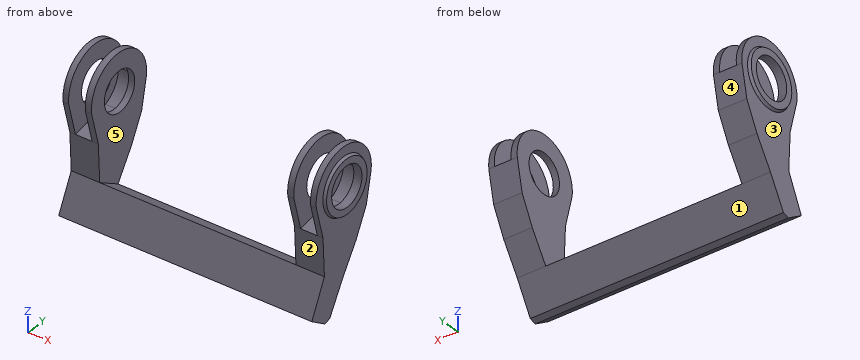
from build123d import *

# Parameters (mm, degrees)
BOSS_EXTRUDE1_DEPTH      = 110.9489018
BOSS_EXTRUDE1_DEPTH_BACK = 110.9489018
BOSS_EXTRUDE2_DEPTH      = 32.209994
CUT_EXTRUDE1_DEPTH       = 18.876772
CUT_EXTRUDE2_DEPTH       = 416.307857918
CUT_EXTRUDE2_DEPTH_BACK  = 416.307857918
SKETCH5_R                = 22.292778643


with BuildPart() as part:
    # Sketch1 → Boss-Extrude1 (new, two sides: drawn at the far end of the back side and taken through both)
    with BuildSketch(Plane(origin=(0, 0, 0), x_dir=(0, 0, -1), z_dir=(1, 0, 0)).offset(-BOSS_EXTRUDE1_DEPTH_BACK)):
        Polygon((6.83514, 301.821342), (21.92401, 328.61631), (55.395622, 309.582058), (57.54243, 302.475138), (45.347128, 283.376878), align=None)
    extrude(amount=BOSS_EXTRUDE1_DEPTH + BOSS_EXTRUDE1_DEPTH_BACK)

    # Sketch2 → Boss-Extrude2 (add)
    with BuildSketch(Plane(origin=(110.9489018, 0, 0), x_dir=(0, 0, -1), z_dir=(1, 0, 0))):
        with BuildLine():
            Line((6.83514, 301.821342), (45.347128, 283.376878))
            Line((45.347128, 283.376878), (57.54243, 302.475138))
            Line((57.54243, 302.475138), (55.395622, 309.582058))
            Line((55.395622, 309.582058), (21.92401, 328.61631))
            Line((21.92401, 328.61631), (-9.123759242, 348.442038748))
            Line((-9.123759242, 348.442038748), (-38.632384, 363.30001))
            Line((-38.632384, 363.30001), (-72.944482, 370.416836))
            ThreePointArc((-72.944482, 370.416836), (-117.407477991, 329.968892479), (-72.634094, 289.8648))
            Line((-72.634094, 289.8648), (-35.4457, 299.743114))
            Line((-35.4457, 299.743114), (6.83514, 301.821342))
        make_face()
    boss_extrude2 = extrude(amount=BOSS_EXTRUDE2_DEPTH)

    # Sketch3 → Cut-Extrude1 (cut)
    with BuildSketch(Plane(origin=(117.9218622, 0, 0), x_dir=(0, 0, -1), z_dir=(1, 0, 0))):
        with BuildLine():
            Line((-72.944482, 370.416836), (-74.851006, 362.67771))
            ThreePointArc((-74.851006, 362.67771), (-56.970321512, 357.844301113), (-44.98594, 343.721436))
            Line((-44.98594, 343.721436), (-35.4457, 299.743114))
            Line((-35.4457, 299.743114), (-71.143283627, 263.85225615))
            Line((-71.143283627, 263.85225615), (-147.020328304, 329.117126747))
            Line((-147.020328304, 329.117126747), (-87.829159197, 385.301513197))
            Line((-87.829159197, 385.301513197), (-72.944482, 370.416836))
        make_face()
    cut_extrude1 = extrude(amount=CUT_EXTRUDE1_DEPTH, mode=Mode.SUBTRACT)

    # Sketch4 → Revolve1 (revolve)
    with BuildSketch(Plane.XY.offset(75.57643), mode=Mode.PRIVATE) as revolve1_sk:
        Polygon((141.481302, 363.150404), (146.090386, 360.588814), (146.090386, 330.870306), (141.481302, 330.870306), align=None)
    revolve1 = revolve(revolve1_sk.sketch.rotate(Axis((146.090386, 330.870306, 75.57643), (-1, 0, 0)), 90), axis=Axis((146.090386, 330.870306, 75.57643), (-1, 0, 0)))

    # Mirror1: Boss-Extrude2, Cut-Extrude1, Revolve1 across plane
    add(boss_extrude2.mirror(Plane(origin=(0, 0, 0), x_dir=(0, 0, 1), z_dir=(1, 0, 0))))
    add(cut_extrude1.mirror(Plane(origin=(0, 0, 0), x_dir=(0, 0, 1), z_dir=(1, 0, 0))), mode=Mode.SUBTRACT)
    add(revolve1.mirror(Plane(origin=(0, 0, 0), x_dir=(0, 0, 1), z_dir=(1, 0, 0))))

    # Sketch5 → Cut-Extrude2 (cut, two sides: drawn at the far end of the back side and taken through both)
    with BuildSketch(Plane(origin=(0, 0, 0), x_dir=(0, 0, -1), z_dir=(1, 0, 0)).offset(-CUT_EXTRUDE2_DEPTH_BACK)):
        with Locations((-75.57643, 330.870306)):
            Circle(SKETCH5_R)
    extrude(amount=CUT_EXTRUDE2_DEPTH + CUT_EXTRUDE2_DEPTH_BACK, mode=Mode.SUBTRACT)


solid = part.part
The model under review builds one solid part; all positions refer to its coordinate system, in mm. Face numbers are marked on the shaded views. A direction names the side the tool comes from. Coordinates: 2 decimals unless noted, no trailing zeros. Loops run counter-clockwise (first coordinate to the right, second up) from the corner with the lowest first, then second, coordinate; pieces in that order, holes last.
(1) Tool access review of the marked faces 1 and 2: name each direction out of +Z, -Z, +X, -X, +Y, -Y from which nothing blocks a thin tool from reaching the whole face with its end or side.
Determined:
face 1: -Z, +X, -X, +Y
face 2: +X, -X, -Y
(2) Insertion check: P1, Ø1, axis at y = 321, z = -32.5, coming from the +X side; P2, Ø4, axis at x = 0, z = -3, coming from the +Y side; P3, Ø8, axis at x = 105, y = 293, coming from the -Z side; P4, Ø1.5, axis at y = 336.5, z = 45.5, coming from the -X side. Each pin has a flat end and moves straight along its axis. Give the tip position at first contact, or say it passes through.
Determined:
P1: stops at x = 143.16
P2: passes through
P3: stops at z = -54.05
P4: stops at x = -145.86
(3) Wall thickness on L1, parallel to X at y = 299, z = 72.5; L2, parallel to X at y = 334.5, z = -2; L3, parallel to X at y = 304, z = 68: over which ranges is each line inside the solid? List them lowest first.
Determined:
L1: x = -143.16 to -136.8, -117.92 to -110.95, 110.95 to 117.92, 136.8 to 143.16
L2: x = -143.16 to -110.95, 110.95 to 143.16
L3: x = -146.09 to -136.8, -117.92 to -110.95, 110.95 to 117.92, 136.8 to 146.09
(4) Draft analysis for pull direction X (two halves, no side actions). For the marked faces 3, 4 and 5, state which applies: +X half, -X half, draft (parallel to the pull), parting line (faces both ways), or undercut.
Determined:
face 3: -X half
face 4: draft
face 5: undercut
(5) Consider section A-A, the plane y = 295. Give the boundary of the cut face in (x, z), plus the area to 3 significant figures.
Determined:
outline: (-143.16, -52.77) - (143.16, -52.77) - (143.16, -21.08) - (-143.16, -21.08) - close; (-143.16, 53.3) - (-136.8, 53.3) - (-136.8, 97.06) - (-143.16, 97.06) - close; (-117.92, 53.3) - (-110.95, 53.3) - (-110.95, 97.06) - (-117.92, 97.06) - close; (110.95, 53.3) - (117.92, 53.3) - (117.92, 97.06) - (110.95, 97.06) - close; (136.8, 53.3) - (143.16, 53.3) - (143.16, 97.06) - (136.8, 97.06) - close
area: 10,200 mm2
(6) Consider section C-C, the plane z = -28.5. Give the boundary of the cut face in (x, y), plus the area to 3 significant figures.
Determined:
outline: (-143.16, 291.45) - (143.16, 291.45) - (143.16, 324.88) - (-143.16, 324.88) - close
area: 9,570 mm2
(7) Consider section B-B, the plane x = -34. Give the boundary of the cut face in (y, z).
Determined:
outline: (283.38, -45.35) - (302.48, -57.54) - (309.58, -55.4) - (328.62, -21.92) - (301.82, -6.84) - close
(8) Consider section D-D, the plane x = 125. Give the boundary of the cut face in (y, z).
Determined:
outline: (283.38, -45.35) - (302.48, -57.54) - (309.58, -55.4) - (328.62, -21.92) - (348.44, 9.12) - (363.3, 38.63) - (370.42, 72.94) - (362.68, 74.85) arc R31.18 cw to (343.72, 44.99) - (299.74, 35.45) - (301.82, -6.84) - close
